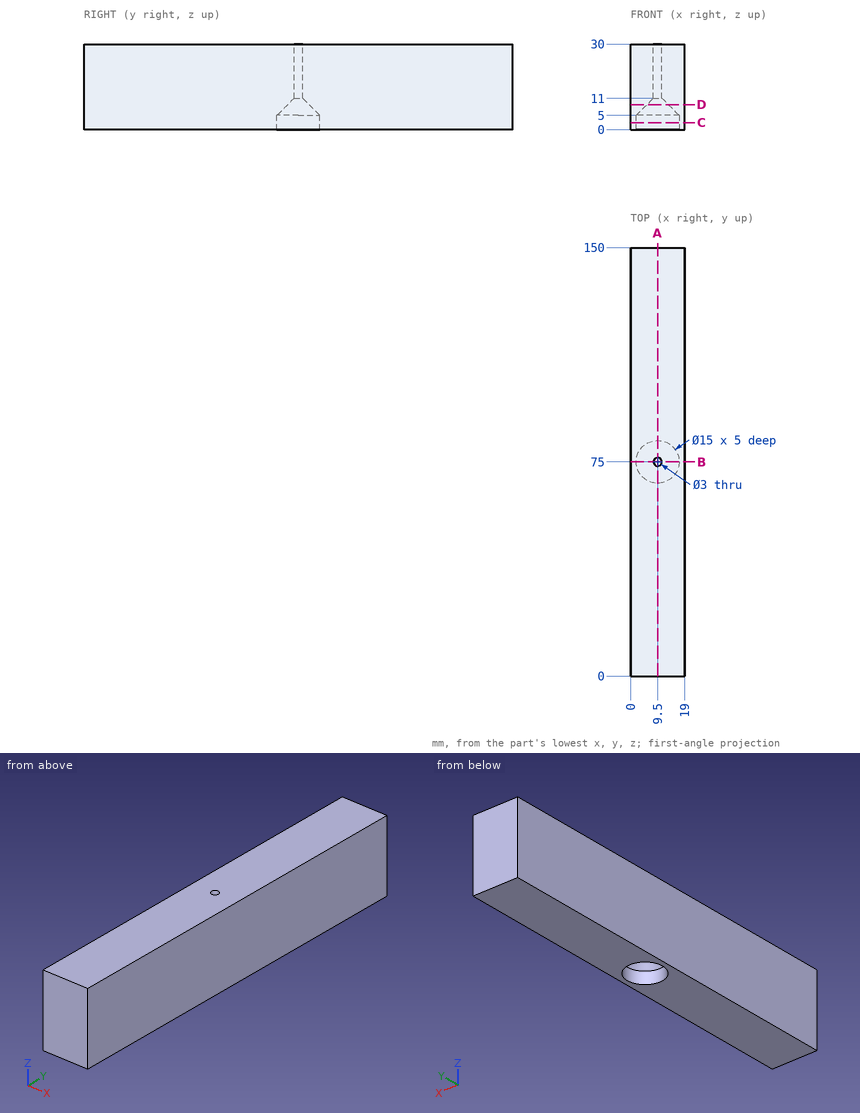
Could you check a few things on this drawing? It's one solid part, dimensions in mm from its lowest x, y, z. Round coordinates to 2 decimals unless told otherwise and drop trailing zeros. Loops run counter-clockwise (first coordinate to the right, second up) from the corner with the lowest first, then second, coordinate; pieces in that order, holes last. Notation, with made-up numbers: M 72,-25 L 104,-25 A35 ccw 104,8 Z; hole C 43,58.5 d9. An arc over 180 degrees is marked long. Write item = value, one per line. Start each with the question number.
(1) Suppose I cut it at A-A on x = 9.5. Write out the boundary of the cut face in (y, z).
(2) I need wall thicknesses on line 1 along Y through (x, z) = (9.5, 24.75); line 2 along Y through (x, z) = (9.5, 1.2); line 3 along X through (y, z) = (75, 2.7). Which ranges of each line are inside material? Lowest first, please.
(3) I'm going to push flat-ended pins straight in: P1, Ø1, axis at x = 3.5, z = 7, coming from the -Y side; P2, Ø3.5, axis at x = 9.5, y = 75, coming from the -Z side. Where does each tip first touch, or does it pass through?
(4) Suppose I cut it at D-D on z = 8.75. Write out the boundary of the cut face in (x, y).
(5) Suppose I cut it at C-C on z = 2.5. Write out the boundary of the cut face in (x, y).
(6) Suppose I cut it at B-B on y = 75. Write out the boundary of the cut face in (x, z).
Answer block:
q1.outline = M 0,0 L 67.5,0 L 67.5,5 L 73.5,11 L 73.5,30 L 0,30 Z; M 76.5,11 L 82.5,5 L 82.5,0 L 150,0 L 150,30 L 76.5,30 Z
q2.line_1 = 0 to 73.5, 76.5 to 150
q2.line_2 = 0 to 67.5, 82.5 to 150
q2.line_3 = 0 to 2, 17 to 19
q3.P1 = 0
q3.P2 = 10.75
q4.outline = M 0,0 L 19,0 L 19,150 L 0,150 Z; hole C 9.5,75 d7.5
q5.outline = M 0,0 L 19,0 L 19,150 L 0,150 Z; hole C 9.5,75 d15
q6.outline = M 0,0 L 2,0 L 2,5 L 8,11 L 8,30 L 0,30 Z; M 11,11 L 17,5 L 17,0 L 19,0 L 19,30 L 11,30 Z
